For this review, take the finished solid that the model builds, in its own axes (mm). Face numbers are marked on the shaded views. A direction names the side the tool comes from. Give positions to 0.01 mm unless a question says otherwise; leave off trailing zeros. Write each loop counter-clockwise with the first axis right and the second up, starting at its lowest first coordinate (ties: lowest second). Pieces come first, ordered by that corner, then holes.
Q1. Machinability: for the marked faces 4, 5 and 6, which of the approach directions +Z, -Z, +X, -X, +Y, -Y give a long, thin tool a straight path to every point of the face, cutting with its end or side? Answer none if there is none.
Q2. We need section A-A (y = -21). Write out the cut boundary in (x, z), then the cut area to 3 significant figures.
Q3. Insertion check: P1, Ø23.5, axis at x = 78.5, z = 44, coming from the -Y side; P2, Ø12, axis at y = -14, z = 41, coming from the -X side; P3, Ø2, axis at y = 5, z = 7, coming from the +X side; P4, Ø12, axis at x = 74.5, y = 1.5, coming from the +Z side. Each pin has a flat end and moves straight along its axis. Give the tip position at first contact, or say it passes through.
Q4. We need section C-C (x = 70). Write out the cut boundary in (y, z).
Q5. Mouldability with a two-part tool opening along X and no side actions: class the marked faces 1, 2 and 3 as released by +X, released by -X, zero draft, split by the parting line, or undercut.
Q6. For line 1 (Z direction, x = 30, y = -21); line 2 (Y direction, x = 86.5, z = 3); line 3 (X direction, y = -25.5, z = 54.5), list the stretches that pass through material, from the lowest coordinate up.
Q7. We need section D-D (z = 51.5). Write out the cut boundary in (x, y).
Q8. We need section B-B (z = 42.5). Write out the cut boundary in (x, y).
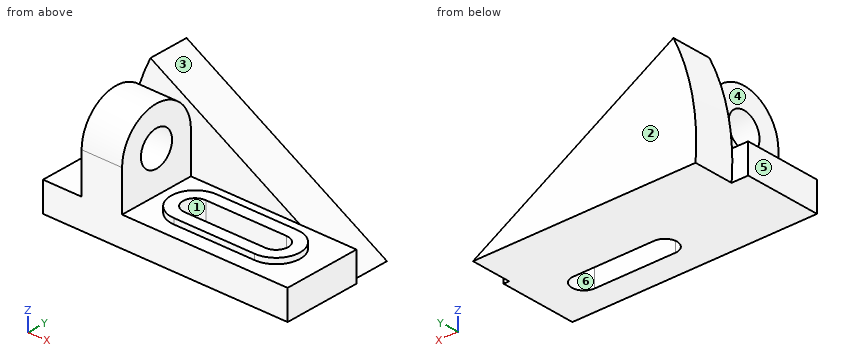
```python
from build123d import *

# Parameters (mm, degrees)
F1_DEPTH  = 42
F2_R      = 9.5
F3_DEPTH  = 43.001
F5_DEPTH  = 43.001
F7_DEPTH  = 3
F9_DEPTH  = 19.001
F11_DEPTH = 22


with BuildPart() as f1:
    # F0 (on Front) → F1 (new body)
    with BuildSketch(Plane.XZ):
        Polygon((0, 16), (0, 0), (133, 0), (133, 16), (43, 16), (43, 60), (21, 60), (21, 16), align=None)
    extrude(amount=F1_DEPTH)

    # F2 (on face) → F3 (cut, through all)
    with BuildSketch(Plane.YZ.offset(43)):
        with Locations((-21, 38)):
            Circle(F2_R)
    extrude(amount=-F3_DEPTH, mode=Mode.SUBTRACT)

    # F4 (on face) → F5 (cut, through all)
    with BuildSketch(Plane.YZ.offset(43)):
        with BuildLine():
            Line((-42, 60), (-42, 38))
            ThreePointArc((-42, 38), (-21, 59), (0, 38))
            Line((0, 38), (0, 60))
            Line((0, 60), (-42, 60))
        make_face()
    extrude(amount=-F5_DEPTH, mode=Mode.SUBTRACT)

    # F6 (on face) → F7 (join)
    with BuildSketch(Plane.XY.offset(16)):
        with BuildLine():
            Line((108, -8), (64, -8))
            ThreePointArc((64, -8), (51, -21), (64, -34))
            Line((64, -34), (108, -34))
            ThreePointArc((108, -34), (121, -21), (108, -8))
        make_face()
    extrude(amount=F7_DEPTH)

    # F8 (on face) → F9 (cut, through all)
    with BuildSketch(Plane.XY.offset(19)):
        with BuildLine():
            Line((108, -14.5), (64, -14.5))
            ThreePointArc((64, -14.5), (57.5, -21), (64, -27.5))
            Line((64, -27.5), (108, -27.5))
            ThreePointArc((108, -27.5), (114.5, -21), (108, -14.5))
        make_face()
    extrude(amount=-F9_DEPTH, mode=Mode.SUBTRACT)

    # F10 (on face) → F11 (join)
    with BuildSketch(Plane(origin=(0, 0, 0), x_dir=(-1, 0, 0), z_dir=(0, 1, 0))):
        with BuildLine():
            Line((-21, 62.931179), (-130, 0))
            Line((-130, 0), (-9, 0))
            ThreePointArc((-9, 0), (-10.759382, 32.27421), (-21, 62.931179))
        make_face()
    extrude(amount=F11_DEPTH)


solid = f1.part
```
Computed:
1. face 4: +Z, -X, -Y
1. face 5: +Z, -Z, -X, +Y, -Y
1. face 6: +Z, -Z
2. outline: (0, 0) - (57.5, 0) - (57.5, 19) - (51, 19) - (51, 16) - (43, 16) - (43, 28.5) - (21, 28.5) - (21, 16) - (0, 16) - close; (21, 47.5) - (43, 47.5) - (43, 59) - (21, 59) - close; (114.5, 0) - (133, 0) - (133, 16) - (121, 16) - (121, 19) - (114.5, 19) - close
2. area: 1,780 mm2
3. P1: passes through
3. P2: stops at x = 21
3. P3: stops at x = 119.61
3. P4: stops at z = 35.51
4. outline: (-42, 0) - (-27.5, 0) - (-27.5, 19) - (-34, 19) - (-34, 16) - (-42, 16) - close; (-14.5, 0) - (22, 0) - (22, 34.64) - (0, 34.64) - (0, 16) - (-8, 16) - (-8, 19) - (-14.5, 19) - close
5. face 1: undercut
5. face 2: zero draft
5. face 3: released by +X
6. line 1: z = 0 to 28.5, 47.5 to 59
6. line 2: y = -42 to -27.5, -14.5 to 22
6. line 3: x = 21 to 43
7. outline: (16.1, 0) - (40.8, 0) - (40.8, 22) - (16.1, 22) - close; (21, -37.09) - (43, -37.09) - (43, -4.91) - (21, -4.91) - close
8. outline: (13.17, 0) - (56.39, 0) - (56.39, 22) - (13.17, 22) - close; (21, -41.51) - (43, -41.51) - (43, -29.37) - (21, -29.37) - close; (21, -12.63) - (43, -12.63) - (43, -0.49) - (21, -0.49) - close
